```python
from build123d import *

# Parameters (mm, degrees)
F0_W           = 152.4
F0_H           = 120.65
F1_DEPTH       = 12.7
F3_D           = 2.54
F3_CSINK_D     = 6.604
F3_CSINK_ANGLE = 90
F5_DEPTH       = 12.701


with BuildPart() as f1:
    # F0 (on Front) → F1 (new body)
    with BuildSketch(Plane.XZ):
        with Locations((0, 3.175)):
            Rectangle(F0_W, F0_H)
    extrude(amount=F1_DEPTH)

    # F3 (through all)
    with Locations(Plane.XZ.offset(12.7)):
        with Locations((-69.85, 50.8), (-69.85, -31.75), (-44.45, -50.8), (44.45, -50.8), (69.85, -31.75), (69.85, 50.8)):
            CounterSinkHole(F3_D / 2, F3_CSINK_D / 2, counter_sink_angle=F3_CSINK_ANGLE)

    # F4 (on face) → F5 (cut, through all)
    with BuildSketch(Plane.XZ.offset(12.7)):
        with BuildLine():
            Line((0, 53.34), (-16, 53.34))
            ThreePointArc((-16, 53.34), (-28.7, 40.64), (-16, 27.94))
            Line((-16, 27.94), (0, 27.94))
            Line((0, 27.94), (16, 27.94))
            ThreePointArc((16, 27.94), (28.7, 40.64), (16, 53.34))
            Line((16, 53.34), (0, 53.34))
        make_face()
    extrude(amount=-F5_DEPTH, mode=Mode.SUBTRACT)


solid = f1.part
```
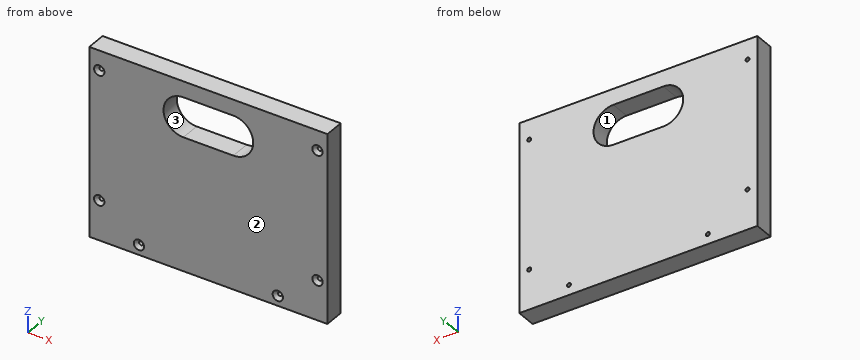
The listing builds one solid part. Answer for the finished solid, in the listing's coordinates (mm). Face numbers are marked on the shaded views. Round coordinates to 2 decimals unless told otherwise and drop trailing zeros. Loops run counter-clockwise (first coordinate to the right, second up) from the corner with the lowest first, then second, coordinate; pieces in that order, holes last. Notation, with made-up numbers: (-32.75, 33) - (3.25, 33) arc R18 ccw to (3.25, 58) - close; hole circle Ø1 at (-6.75, 61). An arc over 180 degrees is marked (long way). Return JSON: item names as keys, results as strings. Group by question number.
1. Each of these flat-tipped pins is pushed along its axis until it touches: P1, Ø3.5, axis at x = 44.45, z = -50.8, coming from the +Y side; P2, Ø2, axis at x = -69.85, z = 50.8, coming from the +Y side. Where does it stop, or does it pass through?
2. The mould has two halves that part along Z. Classify the marked faces 1, 2 and 3: pulls with the +Z half, pulls with the -Z half, needs draft (parallel to the pull), parting line crosses it, or undercut.
3. The part is cut by section C-C on z = 31. Determine the outline of the cut face in (x, y), then the cut area to 3 significant figures.
4. The part is cut by section A-A on y = -4.25. Determine the outline of the cut face in (x, z), then the cut area to 3 significant figures.
5. The part is cut by section B-B on x = -25.5. Determine the outline of the cut face in (y, z).
6. Consider probe 1 along Z at (x, y) = (-69.85, -6.25); probe 2 along X at (y, z) = (-8.25, -50.8); probe 3 along X at (y, z) = (-3.5, -31.75). Determine where each line is inside the solid, lowest interval first.
Resolved:
{
 "1": {"P1": "stops at y = 0", "P2": "passes through"},
 "2": {"face 1": "undercut", "face 2": "needs draft", "face 3": "undercut"},
 "3": {"outline": "(-76.2, -12.7) - (-24.27, -12.7) - (-24.27, 0) - (-76.2, 0) - close; (24.27, -12.7) - (76.2, -12.7) - (76.2, 0) - (24.27, 0) - close", "area": "1,320 mm²"},
 "4": {"outline": "(-76.2, -57.15) - (76.2, -57.15) - (76.2, 63.5) - (-76.2, 63.5) - close; hole circle Ø2.54 at (-69.85, -31.75); hole circle Ø2.54 at (-69.85, 50.8); hole circle Ø2.54 at (-44.45, -50.8); hole (-16, 27.94) - (16, 27.94) arc R12.7 ccw to (16, 53.34) - (-16, 53.34) arc R12.7 ccw to start; hole circle Ø2.54 at (44.45, -50.8); hole circle Ø2.54 at (69.85, -31.75); hole circle Ø2.54 at (69.85, 50.8)", "area": "17,000 mm²"},
 "5": {"outline": "(-12.7, -57.15) - (0, -57.15) - (0, 32.21) - (-12.7, 32.21) - close; (-12.7, 49.07) - (0, 49.07) - (0, 63.5) - (-12.7, 63.5) - close"},
 "6": {"probe 1": "z = -57.15 to -33.02, -30.48 to 49.53, 52.07 to 63.5", "probe 2": "x = -76.2 to -45.72, -43.18 to 43.18, 45.72 to 76.2", "probe 3": "x = -76.2 to -71.12, -68.58 to 68.58, 71.12 to 76.2"}
}
